Geometry check sheet. Reference: the model listing, model coordinates, mm. Face numbers are marked on the shaded views. Round coordinates to 2 decimals unless told otherwise and drop trailing zeros. Order: outer loops, then holes, each group sorted by start corner. A loop starts at its lowest first (then second) coordinate and runs counter-clockwise, first axis right, second up. Notation, with made-up numbers: (21, -29) -> (40, -29) arc R30 ccw to (40, 3) -> close; hole circle Ø5 at (-9, 56). An arc over 180 degrees is marked (long way). Answer as a JSON object with one key per item and string values. Group by question number.
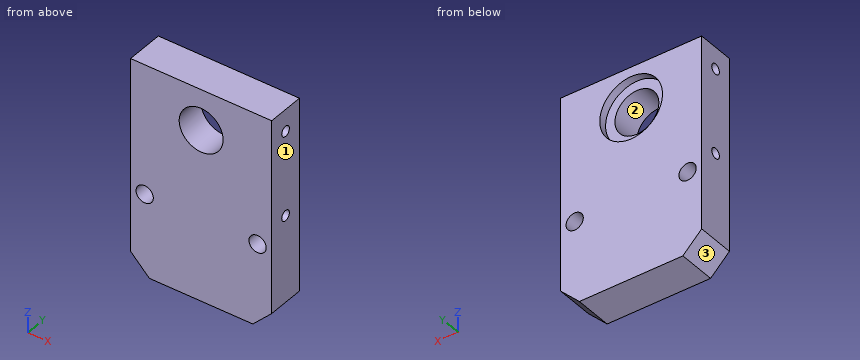
from build123d import *

# Parameters (mm, degrees)
SKETCH1_R             = 2.75
SKETCH1_R_2           = 7
BOSS_EXTRUDE1_DEPTH   = 12
M4_TAPPED_HOLE1_D     = 3.3
M4_TAPPED_HOLE1_DEPTH = 14
M4_TAPPED_HOLE1_TIP   = 0.991420021
M4_TAPPED_HOLE2_D     = 3.3
M4_TAPPED_HOLE2_DEPTH = 14
M4_TAPPED_HOLE2_TIP   = 0.991420021
SKETCH6_R             = 10
CUT_EXTRUDE1_DEPTH    = 2.5


with BuildPart() as part:
    # Sketch1 → Boss-Extrude1 (new body)
    with BuildSketch(Plane(origin=(0, 0, 0), x_dir=(1, 0, 0), z_dir=(0, 1, 0))):
        Polygon((-16.5, 33.888888889), (-22.5, 27.888888889), (-22.5, -33.888888889), (22.5, -33.888888889), (22.5, 27.888888889), (16.5, 33.888888889), align=None)
        with Locations((-18, 7.611111111)):
            Circle(SKETCH1_R, mode=Mode.SUBTRACT)
        with Locations((18, 7.611111111)):
            Circle(SKETCH1_R, mode=Mode.SUBTRACT)
        with Locations((0, -20.888888889)):
            Circle(SKETCH1_R_2, mode=Mode.SUBTRACT)
    extrude(amount=BOSS_EXTRUDE1_DEPTH)

    # M4 Tapped Hole1
    with Locations(Plane.ZY.offset(22.5)):
        with Locations((-0.111111111, 6), (26.888888889, 6)):
            Hole(M4_TAPPED_HOLE1_D / 2, depth=M4_TAPPED_HOLE1_DEPTH)
            with Locations((0, 0, -(M4_TAPPED_HOLE1_DEPTH + M4_TAPPED_HOLE1_TIP / 2))):  # 118° drill point
                Cone(0, M4_TAPPED_HOLE1_D / 2, M4_TAPPED_HOLE1_TIP, mode=Mode.SUBTRACT)

    # M4 Tapped Hole2
    with Locations(Plane(origin=(22.5, 0, 0), x_dir=(0, 0, -1), z_dir=(1, 0, 0))):
        with Locations((-26.888888889, 6), (0.111111111, 6)):
            Hole(M4_TAPPED_HOLE2_D / 2, depth=M4_TAPPED_HOLE2_DEPTH)
            with Locations((0, 0, -(M4_TAPPED_HOLE2_DEPTH + M4_TAPPED_HOLE2_TIP / 2))):  # 118° drill point
                Cone(0, M4_TAPPED_HOLE2_D / 2, M4_TAPPED_HOLE2_TIP, mode=Mode.SUBTRACT)

    # Sketch6 → Cut-Extrude1 (cut)
    with BuildSketch(Plane(origin=(0, 12, 0), x_dir=(1, 0, 0), z_dir=(0, 1, 0))):
        with Locations((0, -20.888888889)):
            Circle(SKETCH6_R)
    extrude(amount=-CUT_EXTRUDE1_DEPTH, mode=Mode.SUBTRACT)


solid = part.part
Item 1: Sectioned sample at B-B, the plane x = -18. Enter the section's corners in (y, z).
Item 2: Sectioned sample at A-A, the plane x = 0. Enter the section's corners in (y, z).
Item 3: Thickness scan on L1, parallel to Z at x = 14, y = 6; L2, parallel to Z at x = 0, y = 10.5; L3, parallel to X at y = 1.5, z = -7. Record the ranges inside material, lowest first.
Item 4: Depth check by flat-ended pin: pin 1 Ø3.5 at (x, z) = (18, -7.61) entering from +Y; pin 2 Ø2 at (y, z) = (6, 26.89) entering from +X; pin 3 Ø3 at (y, z) = (6, 26.89) entering from -X. Enter the tip coordinate at first touch or a pass-through.
Item 5: Sectioned sample at C-C, the plane y = 10.5. Enter the section's corners in (x, z).
Item 6: Sectioned sample at D-D, the plane y = 2.5. Enter the section's corners in (x, z), then the cut area to 3 significant figures.
Item 7: Mould release check, pull along Z, two halves, no side actions. Record for the marked faces 1, 2 and 3: pulls with the +Z half, pulls with the -Z half, needs draft (parallel to the pull), parting line crosses it, or undercut.
Result:
{
 "1": {"outline": "(0, -32.39) -> (12, -32.39) -> (12, -10.36) -> (0, -10.36) -> close; (0, -4.86) -> (12, -4.86) -> (12, 33.89) -> (0, 33.89) -> close; hole circle Ø3.3 at (6, -0.11); hole circle Ø3.3 at (6, 26.89)"},
 "2": {"outline": "(0, -33.89) -> (12, -33.89) -> (12, 10.89) -> (9.5, 10.89) -> (9.5, 13.89) -> (0, 13.89) -> close; (0, 27.89) -> (9.5, 27.89) -> (9.5, 30.89) -> (12, 30.89) -> (12, 33.89) -> (0, 33.89) -> close"},
 "3": {"L1": "z = -33.89 to -1.76, 1.54 to 25.24, 28.54 to 33.89", "L2": "z = -33.89 to 10.89, 30.89 to 33.89", "L3": "x = -22.5 to -20.68, -15.32 to 15.32, 20.68 to 22.5"},
 "4": {"pin 1": "passes through", "pin 2": "stops at x = 8.11", "pin 3": "stops at x = -8.41"},
 "5": {"outline": "(-22.5, -27.89) -> (-16.5, -33.89) -> (16.5, -33.89) -> (22.5, -27.89) -> (22.5, 33.89) -> (-22.5, 33.89) -> close; hole circle Ø5.5 at (-18, -7.61); hole circle Ø20 at (0, 20.89); hole circle Ø5.5 at (18, -7.61)"},
 "6": {"outline": "(-22.5, -27.89) -> (-16.5, -33.89) -> (16.5, -33.89) -> (22.5, -27.89) -> (22.5, 33.89) -> (-22.5, 33.89) -> close; hole circle Ø5.5 at (-18, -7.61); hole circle Ø14 at (0, 20.89); hole circle Ø5.5 at (18, -7.61)", "area": "2,810 mm2"},
 "7": {"face 1": "needs draft", "face 2": "undercut", "face 3": "pulls with the -Z half"}
}
